The model under review builds one solid part; all positions refer to its coordinate system, in mm. Face numbers are marked on the shaded views. A direction names the side the tool comes from. Round coordinates to 2 decimals unless told otherwise and drop trailing zeros. Write each loop counter-clockwise with the first axis right and the second up, starting at its lowest first coordinate (ties: lowest second). Pieces come first, ordered by that corner, then holes. Notation, with made-up numbers: M -34.5,75 L -25.5,75 A23 cw -25.5,102 Z; hole C 21.25,-0.75 d11. An arc over 180 degrees is marked long. One line per item, written item: value. Start each with the question number.
1) For P1, Ø1.6, axis at y = 4.5, z = 0.5, coming from the -X side; P2, Ø0.8, axis at x = -1.5, z = -0.5, coming from the -Y side; P3, Ø2, axis at x = 2.5, z = 2.5, coming from the -Y side, all flat-tipped, find the tip position at first contact; note any pin that passes through.
2) Take a section at D-D, the plane x = -4.5. Write out the cut boundary in (y, z).
3) Take a section at A-A, the plane y = 0. Write out the cut boundary in (x, z), and give its area (3 significant figures).
4) Take a section at C-C, the plane z = -3.75. Write out the cut boundary in (x, y).
5) Tool access review of the marked faces 4, 5, 6 and 7: name each direction out of +Z, -Z, +X, -X, +Y, -Y from which nothing blocks a thin tool from reaching the whole face with its end or side.
6) Wall thickness on probe 1 along X at (y, z) = (-4, -1.75); probe 2 along X at (y, z) = (-4.5, 2.25); probe 3 along Z at (x, y) = (-4.25, -1.75): over which ranges is each line inside the solid? List them lowest first.
7) Take a section at B-B, the plane x = 0. Write out the cut boundary in (y, z).
8) Mouldability with a two-part tool opening along Y and no side actions: class the marked faces 1, 2 and 3 as +Y half, -Y half, draft (parallel to the pull), parting line (faces both ways), or undercut.
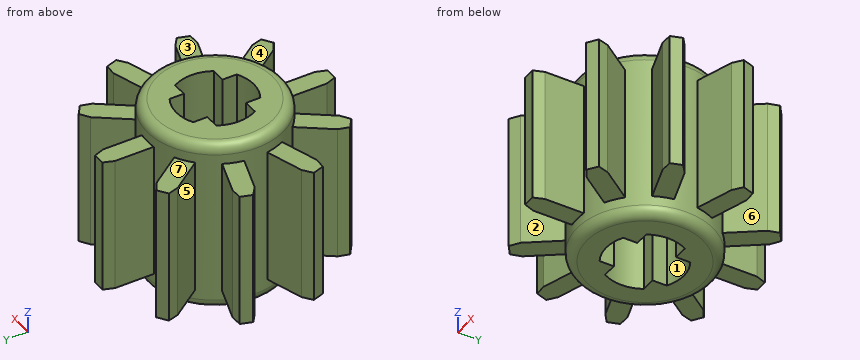
from build123d import *

# Parameters (mm, degrees)
SKETCH1_R           = 3.5
SKETCH1_R_2         = 2
BOSS_EXTRUDE1_DEPTH = 4.5
BOSS_EXTRUDE2_DEPTH = 3.5
CIRPATTERN1_COUNT   = 10
FILLET1_R           = 0.5


with BuildPart() as part:
    # Sketch1 → Boss-Extrude1 (new body, symmetric)
    with BuildSketch(Plane.XY):
        Circle(SKETCH1_R)
        Circle(SKETCH1_R_2, mode=Mode.SUBTRACT)
        with BuildLine():
            Line((1, -1), (1, -1.732050808))
            ThreePointArc((1, -1.732050808), (1.414213562, -1.414213562), (1.732050808, -1))
            Line((1.732050808, -1), (1, -1))
        make_face()
        with BuildLine():
            ThreePointArc((-1.732050808, -1), (-1.414213562, -1.414213562), (-1, -1.732050808))
            Line((-1, -1.732050808), (-1, -1))
            Line((-1, -1), (-1.732050808, -1))
        make_face()
        with BuildLine():
            Line((-1.732050808, 1), (-1, 1))
            Line((-1, 1), (-1, 1.732050808))
            ThreePointArc((-1, 1.732050808), (-1.414213562, 1.414213562), (-1.732050808, 1))
        make_face()
        with BuildLine():
            Line((1, 1.732050808), (1, 1))
            Line((1, 1), (1.732050808, 1))
            ThreePointArc((1.732050808, 1), (1.414213562, 1.414213562), (1, 1.732050808))
        make_face()
    extrude(amount=BOSS_EXTRUDE1_DEPTH, both=True)

    # Sketch2 → Boss-Extrude2 (add, symmetric)
    with BuildSketch(Plane.XY):
        with BuildLine():
            Line((-0.5, 3.464101615), (-0.5, 5.464101615))
            Line((-0.5, 5.464101615), (-0.304948939, 6))
            Line((-0.304948939, 6), (0.304948939, 6))
            Line((0.304948939, 6), (0.5, 5.464101615))
            Line((0.5, 5.464101615), (0.5, 3.464101615))
            ThreePointArc((0.5, 3.464101615), (0, 3.5), (-0.5, 3.464101615))
        make_face()
    boss_extrude2 = extrude(amount=BOSS_EXTRUDE2_DEPTH, both=True)

    # CirPattern1: Boss-Extrude2 ×10 about axis
    cirpattern1_axis = Axis((0, 0, 0), (0, 0, 1))
    for i in range(1, CIRPATTERN1_COUNT):
        add(boss_extrude2.rotate(cirpattern1_axis, i * 360 / CIRPATTERN1_COUNT))

    # Fillet1
    fillet1_edges = [part.edges().sort_by_distance(p)[0] for p in [
        (-3.5, 0, -4.5),
        (-3.5, 0, 4.5),
    ]]
    fillet(fillet1_edges, radius=FILLET1_R)


solid = part.part
Checked values:
1. P1: stops at x = -3.77
1. P2: stops at y = -3.47
1. P3: stops at y = -5.03
2. outline: M -1.99,-3.5 L -0.94,-3.5 L -0.94,3.5 L -1.99,3.5 Z; M 0.94,-3.5 L 1.99,-3.5 L 1.99,3.5 L 0.94,3.5 Z
3. outline: M -3.5,-4 A0.5 ccw -3,-4.5 L -2,-4.5 L -2,4.5 L -3,4.5 A0.5 ccw -3.5,4 Z; M 2,-4.5 L 3,-4.5 A0.5 ccw 3.5,-4 L 3.5,4 A0.5 ccw 3,4.5 L 2,4.5 Z
3. area: 26.8 mm2
4. outline: C 0,0 d7; hole M -1.73,-1 L -1,-1 L -1,-1.73 A2 ccw 1,-1.73 L 1,-1 L 1.73,-1 A2 ccw 1.73,1 L 1,1 L 1,1.73 A2 ccw -1,1.73 L -1,1 L -1.73,1 A2 ccw Z
5. face 4: +Z, +X, -Y
5. face 5: +Z, -Z, -X
5. face 6: +Z, -Z, +X
5. face 7: +Z, -X, +Y
6. probe 1: x = -3.52 to -2.29, -0.5 to 0.5, 2.29 to 3.52
6. probe 2: x = -3.72 to -2.65, -0.5 to 0.5, 2.65 to 3.72
6. probe 3: z = -3.5 to 3.5
7. outline: M -6,-3.5 L -3.5,-3.5 L -3.5,-4 A0.5 ccw -3,-4.5 L -2,-4.5 L -2,4.5 L -3,4.5 A0.5 ccw -3.5,4 L -3.5,3.5 L -6,3.5 Z; M 2,-4.5 L 3,-4.5 A0.5 ccw 3.5,-4 L 3.5,-3.5 L 6,-3.5 L 6,3.5 L 3.5,3.5 L 3.5,4 A0.5 ccw 3,4.5 L 2,4.5 Z
8. face 1: undercut
8. face 2: -Y half
8. face 3: draft
